from build123d import *

# Parameters (mm, degrees)
F0_W          = 80
F0_H          = 102
F1_DEPTH      = 36
F2_W          = 100
F2_H          = 20
F3_DEPTH      = 72
F4_R          = 28
F5_DEPTH      = 8
F6_R          = 31
F6_R_2        = 19
F7_DEPTH      = 16
F7_DEPTH_BACK = 80
F8_DEPTH      = 80.001
F9_R          = 32
F10_DEPTH     = 45.001


# Not quite as in the source:
# - a pattern or mirror of a feature is missing from the dataset's text; its kind, count and spacing are read off the source's solid


with BuildPart() as f1:
    # F0 (on Right) → F1 (new body, symmetric)
    with BuildSketch(Plane.YZ):
        Rectangle(F0_W, F0_H)
    extrude(amount=F1_DEPTH, both=True)

    # F2 (on face) → F3 (join, through all)
    with BuildSketch(Plane.YZ.offset(36)):
        with Locations((-90, -16)):
            Rectangle(F2_W, F2_H)
    extrude(amount=-F3_DEPTH)

    # F4 (on face) → F5 (cut)
    with BuildSketch(Plane.YZ.offset(36)):
        with Locations((0, -16)):
            Circle(F4_R)
    f5 = extrude(amount=-F5_DEPTH, mode=Mode.SUBTRACT)

    # F5_copies: F5 across plane
    add(f5.mirror(Plane(origin=(0, 0, 0), x_dir=(0, 0, -1), z_dir=(-1, 0, 0))), mode=Mode.SUBTRACT)

    # F6 (on face) → F7 (join, two sides)
    with BuildSketch(Plane.XZ.offset(40)) as f7_sk:
        with Locations((0, 42)):
            Circle(F6_R)
        with Locations((0, 42)):
            Circle(F6_R_2, mode=Mode.SUBTRACT)
    extrude(amount=F7_DEPTH)
    extrude(f7_sk.sketch, amount=-F7_DEPTH_BACK)

    # F8 (cut, through all): a face of the model
    f8_faces = [f1.faces().sort_by_distance(p)[0] for p in [
        (0, -40, 38.5131332961),
    ]]
    extrude(f8_faces, amount=-F8_DEPTH, mode=Mode.SUBTRACT)

    # F9 (on face) → F10 (cut, through all)
    with BuildSketch(Plane.XY.offset(-6)):
        with Locations((0, -90)):
            Circle(F9_R)
    extrude(amount=-F10_DEPTH, mode=Mode.SUBTRACT)


solid = f1.part
Geometry: final body of the model. Coordinates: model frame, mm. A direction names the side the tool comes from. Coordinates: 2 decimals unless noted, no trailing zeros. Order: outer loops, then holes, each group sorted by start corner. A loop starts at its lowest first (then second) coordinate and runs counter-clockwise, first axis right, second up. Notation, with made-up numbers: M 47,79 L 56,79 A22 ccw 56,90 Z; hole C -27.5,-23.75 d7. An arc over 180 degrees is marked long. One line per question, with ' | ' between items. Start each with the question number.
Item 1: Set-up query: faces 4 (the flat face through (33, -91, -26)), 5 (the flat face through (28, 0, -16)), 6 (the flat face through (-33, -1, 51)), 7 (the flat face through (-28, 0, -16)), 8 (the flat face through (33, -1, 51)). Return all of +Z, -Z, +X, -X, +Y, -Y with unobstructed straight access to the full face (end or side cutting, diameter ignored); none if empty.
Item 2: Draft query along Z for faces 1 (the flat face through (1, -140, -16)), 2 (the flat face through (1, -1, -51)), 3 (the flat face through (33, -91, -6)). Return one class per face: released by +Z, released by -Z, zero draft, split by the parting line, or undercut.
Item 3: Cut plane C-C, the plane z = 42. Return the cut outline in (x, y), then the cut area to 3 significant figures.
Item 4: Ray query, probe 1 along Z at (x, y) = (0, -3.5); probe 2 along X at (y, z) = (-30.5, 42); probe 3 along Y at (x, z) = (0, -16.5). Return the intervals inside material, ascending. Write a range as [from, to].
Item 5: Cut plane A-A, the plane y = -90. Return the cut outline in (x, z).
Item 6: Cut plane B-B, the plane x = 0. Return the cut outline in (y, z).
Item 7: Pin query (flat end, axial travel): pin 1 Ø2 at (y, z) = (-15.5, 53) entering from -X; pin 2 Ø8 at (x, y) = (28.5, -2.5) entering from +Z; pin 3 Ø5 at (x, y) = (23.5, 4) entering from +Z. Return the tip coordinate at first contact, or that it passes through.
Item 8: Cut plane D-D, the plane y = -42. Return the cut outline in (x, z).
A:
1) face 4: -Z, +X, -X, -Y | face 5: +X | face 6: +Z, -X, +Y, -Y | face 7: -X | face 8: +Z, +X, +Y, -Y
2) face 1: zero draft | face 2: released by -Z | face 3: undercut
3) outline: M -36,-40 L -31,-40 L -31,-56 L -19,-56 L -19,40 L -36,40 Z; M 19,-56 L 31,-56 L 31,-40 L 36,-40 L 36,40 L 19,40 Z | area: 3,100 mm2
4) probe 1: z = [-51, 23], [61, 73] | probe 2: x = [-36, -19], [19, 36] | probe 3: y = [-140, -122], [-58, 40]
5) outline: M -36,-26 L -32,-26 L -32,-6 L -36,-6 Z; M 32,-26 L 36,-26 L 36,-6 L 32,-6 Z
6) outline: M -140,-26 L -122,-26 L -122,-6 L -140,-6 Z; M -58,-26 L -40,-26 L -40,-51 L 40,-51 L 40,23 L -56,23 L -56,11 L -40,11 L -40,-6 L -58,-6 Z; M -56,61 L 40,61 L 40,73 L -56,73 Z
7) pin 1: stops at x = -29.34 | pin 2: stops at z = 60.99 | pin 3: stops at z = 64.8
8) outline: M -36,-26 L 36,-26 L 36,-6 L -36,-6 Z; C 0,42 d62; hole C 0,42 d38
